Part model, mm, in its own coordinate system. Face numbers are marked on the shaded views. A direction names the side the tool comes from. Round coordinates to 2 decimals unless told otherwise and drop trailing zeros. Loops run counter-clockwise (first coordinate to the right, second up) from the corner with the lowest first, then second, coordinate; pieces in that order, holes last. Notation, with made-up numbers: (86, 89) -> (141, 89) arc R10 cw to (141, 98) -> close; hole circle Ø5 at (48, 74). An arc over 180 degrees is marked (long way). Answer as CSV lines item,"result".
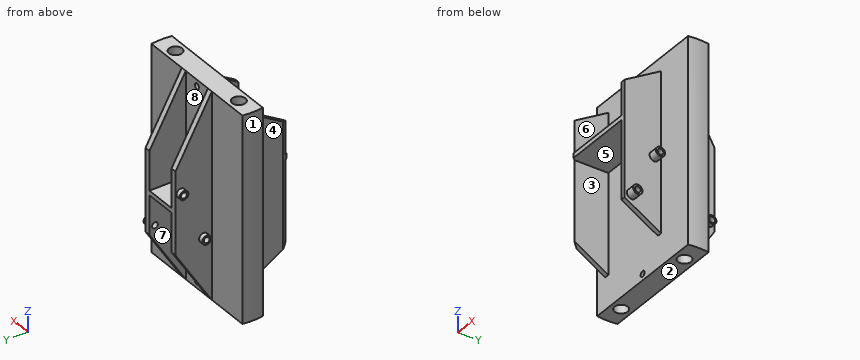
from build123d import *

# Parameters (mm, degrees)
SKETCH1_R            = 5.715
SKETCH1_R_2          = 3.683
BOSS_EXTRUDE2_DEPTH  = 114.3
SKETCH2_W            = 3.175
SKETCH2_H            = 45.974
BOSS_EXTRUDE3_DEPTH  = 20.32
SKETCH8_W            = 17.78
SKETCH8_H            = 2.54
BOSS_EXTRUDE6_DEPTH  = 20.32
BOSS_EXTRUDE9_DEPTH  = 20.32
CUT_EXTRUDE5_REACH   = 130.614
SKETCH10_R           = 1.5875
CUT_EXTRUDE6_REACH   = 126.596
SKETCH13_R           = 1.5875
BOSS_EXTRUDE14_DEPTH = 3.175
BOSS_EXTRUDE15_DEPTH = 3.175
BOSS_EXTRUDE16_START = 5.08
SKETCH12_R           = 2.590347575
SKETCH12_R_2         = 1.5875
SKETCH12_R_3         = 2.612210891
BOSS_EXTRUDE16_DEPTH = 5.08
CHAMFER1_SIZE        = 2.54
SKETCH21_R           = 1.6256
CUT_EXTRUDE7_DEPTH   = 5.08
SKETCH22_R           = 1.6256
CUT_EXTRUDE8_DEPTH   = 5.08
BOSS_EXTRUDE17_START = 2.54
SKETCH23_R           = 2.426614549
SKETCH23_R_2         = 1.6256
SKETCH23_R_3         = 2.598483989
BOSS_EXTRUDE17_DEPTH = 2.54
BOSS_EXTRUDE18_START = 2.54
SKETCH24_R           = 2.467964506
SKETCH24_R_2         = 1.6256
SKETCH24_R_3         = 2.533270714
BOSS_EXTRUDE18_DEPTH = 2.54
SKETCH25_R           = 48.771557558
SKETCH25_R_2         = 36.957
CUT_EXTRUDE9_DEPTH   = 124.263624906
CUT_EXTRUDE10_DEPTH  = 129.148442846


with BuildPart() as part:
    # Sketch1 → Boss-Extrude2 (new body)
    # profile 1 of 8: a face of its own
    with BuildSketch(Plane.XY):
        with BuildLine():
            Line((25.4, 5.715), (-25.4, 5.715))
            ThreePointArc((-25.4, 5.715), (-21.358884746, 4.041115254), (-19.685, 0))
            Line((-19.685, 0), (19.685, 0))
            ThreePointArc((19.685, 0), (21.358884746, 4.041115254), (25.4, 5.715))
        make_face()
    # profile 2 of 8: a face of its own
    with BuildSketch(Plane.XY):
        with Locations((-25.4, 0)):
            Circle(SKETCH1_R)
        with Locations((-25.4, 0)):
            Circle(SKETCH1_R_2, mode=Mode.SUBTRACT)
    # profile 3 of 8: a face of its own
    with BuildSketch(Plane.XY):
        with Locations((25.4, 0)):
            Circle(SKETCH1_R)
        with Locations((25.4, 0)):
            Circle(SKETCH1_R_2, mode=Mode.SUBTRACT)
    # profile 4 of 8: a face of its own
    with BuildSketch(Plane.XY):
        with BuildLine():
            ThreePointArc((-31.115, 0), (-29.441115254, 4.041115254), (-25.4, 5.715))
            Line((-25.4, 5.715), (-37.668936473, 5.715))
            ThreePointArc((-37.668936473, 5.715), (-37.992081278, 2.865616895), (-38.1, 0))
            Line((-38.1, 0), (-31.115, 0))
        make_face()
    # profile 5 of 8: a face of its own
    with BuildSketch(Plane.XY):
        with BuildLine():
            Line((37.668936473, 5.715), (25.4, 5.715))
            ThreePointArc((25.4, 5.715), (29.441115254, 4.041115254), (31.115, 0))
            Line((31.115, 0), (38.1, 0))
            ThreePointArc((38.1, 0), (37.992081278, 2.865616895), (37.668936473, 5.715))
        make_face()
    # profile 6 of 8: a face of its own
    with BuildSketch(Plane.XY):
        with BuildLine():
            Line((38.1, 0), (31.115, 0))
            ThreePointArc((31.115, 0), (29.441115254, -4.041115254), (25.4, -5.715))
            Line((25.4, -5.715), (37.668936473, -5.715))
            ThreePointArc((37.668936473, -5.715), (37.992081278, -2.865616895), (38.1, 0))
        make_face()
    # profile 7 of 8: a face of its own
    with BuildSketch(Plane.XY):
        with BuildLine():
            Line((19.685, 0), (-19.685, 0))
            ThreePointArc((-19.685, 0), (-21.358884746, -4.041115254), (-25.4, -5.715))
            Line((-25.4, -5.715), (25.4, -5.715))
            ThreePointArc((25.4, -5.715), (21.358884746, -4.041115254), (19.685, 0))
        make_face()
    # profile 8 of 8: a face of its own
    with BuildSketch(Plane.XY):
        with BuildLine():
            ThreePointArc((-25.4, -5.715), (-29.441115254, -4.041115254), (-31.115, 0))
            Line((-31.115, 0), (-38.1, 0))
            ThreePointArc((-38.1, 0), (-37.992081278, -2.865616895), (-37.668936473, -5.715))
            Line((-37.668936473, -5.715), (-25.4, -5.715))
        make_face()
    extrude(amount=BOSS_EXTRUDE2_DEPTH)

    # Sketch2 → Boss-Extrude3 (add)
    with BuildSketch(Plane(origin=(0, 5.715, 0), x_dir=(1, 0, 0), z_dir=(0, 1, 0))):
        with Locations((-10.427436473, -54.991)):
            Rectangle(SKETCH2_W, SKETCH2_H)
        with Locations((10.527563527, -54.991)):
            Rectangle(SKETCH2_W, SKETCH2_H)
    extrude(amount=BOSS_EXTRUDE3_DEPTH)

    # Sketch8 → Boss-Extrude6 (add)
    with BuildSketch(Plane(origin=(0, 5.715, 0), x_dir=(1, 0, 0), z_dir=(0, 1, 0))):
        with Locations((0.050063527, -54.991)):
            Rectangle(SKETCH8_W, SKETCH8_H)
    extrude(amount=BOSS_EXTRUDE6_DEPTH)

    # Sketch9 → Boss-Extrude9 (add)
    with BuildSketch(Plane.XZ.offset(5.715)):
        Polygon((12.268936473, 73.66), (12.268936473, 17.78), (14.808936473, 17.78), (14.808936473, 106.68), (12.268936473, 106.68), (12.268936473, 76.2), (-27.508936473, 76.2), (-27.508936473, 106.68), (-30.048936473, 106.68), (-30.048936473, 17.78), (-27.508936473, 17.78), (-27.508936473, 73.66), align=None)
    extrude(amount=BOSS_EXTRUDE9_DEPTH)

    # Sketch10 → Cut-Extrude5 (cut, up to next)
    with BuildSketch(Plane(origin=(14.808936473, 0, 0), x_dir=(0, 0, -1), z_dir=(1, 0, 0)), mode=Mode.PRIVATE) as cut_extrude5_sk1:
        with Locations((-58.42, -9.525)):
            Circle(SKETCH10_R)
    cut_extrude5_tool1 = extrude(cut_extrude5_sk1.sketch, amount=-CUT_EXTRUDE5_REACH, mode=Mode.PRIVATE) & part.part
    # Sketch10 → Cut-Extrude5 (cut, up to next)
    with BuildSketch(Plane(origin=(14.808936473, 0, 0), x_dir=(0, 0, -1), z_dir=(1, 0, 0)), mode=Mode.PRIVATE) as cut_extrude5_sk2:
        with Locations((-33.02, -22.225)):
            Circle(SKETCH10_R)
    cut_extrude5_tool2 = extrude(cut_extrude5_sk2.sketch, amount=-CUT_EXTRUDE5_REACH, mode=Mode.PRIVATE) & part.part
    add(cut_extrude5_tool1.solids().sort_by_distance((14.808936, -9.525, 58.42))[0], mode=Mode.SUBTRACT)
    add(cut_extrude5_tool2.solids().sort_by_distance((14.808936, -22.225, 33.02))[0], mode=Mode.SUBTRACT)

    # Sketch13 → Cut-Extrude6 (cut, up to next)
    with BuildSketch(Plane.XZ.offset(5.715), mode=Mode.PRIVATE) as cut_extrude6_sk1:
        with Locations(Location((0, 110.744, 0), (0, 0, 270))):
            Circle(SKETCH13_R)
    cut_extrude6_tool1 = extrude(cut_extrude6_sk1.sketch, amount=-CUT_EXTRUDE6_REACH, mode=Mode.PRIVATE) & part.part
    # Sketch13 → Cut-Extrude6 (cut, up to next)
    with BuildSketch(Plane.XZ.offset(5.715), mode=Mode.PRIVATE) as cut_extrude6_sk2:
        with Locations(Location((0, 3.556, 0), (0, 0, 270))):
            Circle(SKETCH13_R)
    cut_extrude6_tool2 = extrude(cut_extrude6_sk2.sketch, amount=-CUT_EXTRUDE6_REACH, mode=Mode.PRIVATE) & part.part
    add(cut_extrude6_tool1.solids().sort_by_distance((0, -5.715, 110.744))[0], mode=Mode.SUBTRACT)
    add(cut_extrude6_tool2.solids().sort_by_distance((0, -5.715, 3.556))[0], mode=Mode.SUBTRACT)

    # Sketch18 → Boss-Extrude14 (add)
    with BuildSketch(Plane.ZY.offset(12.014936473)):
        Polygon((77.978, 5.715), (77.978, 26.035), (114.3, 5.715), align=None)
        Polygon((32.004, 26.035), (32.004, 5.715), (0, 5.715), align=None)
    extrude(amount=-BOSS_EXTRUDE14_DEPTH)

    # Sketch19 → Boss-Extrude15 (add)
    with BuildSketch(Plane(origin=(12.115063527, 0, 0), x_dir=(0, 0, -1), z_dir=(1, 0, 0))):
        Polygon((-32.004, 26.035), (0, 5.715), (-32.004, 5.715), align=None)
        Polygon((-77.978, 5.715), (-114.3, 5.715), (-77.978, 26.035), align=None)
    extrude(amount=-BOSS_EXTRUDE15_DEPTH)

    # Sketch12 → Boss-Extrude16 (add)
    # profile 1 of 2: a face of its own
    with BuildSketch(Plane(origin=(14.808936473, 0, 0), x_dir=(0, 0, -1), z_dir=(1, 0, 0)).offset(BOSS_EXTRUDE16_START)):
        with Locations(Location((-58.42, -9.525, 0), (0, 0, 180))):
            Circle(SKETCH12_R)
        with Locations((-58.42, -9.525)):
            Circle(SKETCH12_R_2, mode=Mode.SUBTRACT)
    # profile 2 of 2: a face of its own
    with BuildSketch(Plane(origin=(14.808936473, 0, 0), x_dir=(0, 0, -1), z_dir=(1, 0, 0)).offset(BOSS_EXTRUDE16_START)):
        with Locations(Location((-33.02, -22.225, 0), (0, 0, 180))):
            Circle(SKETCH12_R_3)
        with Locations((-33.02, -22.225)):
            Circle(SKETCH12_R_2, mode=Mode.SUBTRACT)
    extrude(amount=-BOSS_EXTRUDE16_DEPTH)

    # Chamfer1
    chamfer1_edges = [part.edges().sort_by_distance(p)[0] for p in [
        (-30.048936473, -26.035, 62.23),
    ]]
    chamfer(chamfer1_edges, length=CHAMFER1_SIZE)

    # Sketch21 → Cut-Extrude7 (cut)
    with BuildSketch(Plane.ZY.offset(12.014936473)):
        with Locations((65.125187458, 23.037602192)):
            Circle(SKETCH21_R)
        with Locations((35.915187458, 10.337602192)):
            Circle(SKETCH21_R)
    extrude(amount=-CUT_EXTRUDE7_DEPTH, mode=Mode.SUBTRACT)

    # Sketch22 → Cut-Extrude8 (cut)
    with BuildSketch(Plane(origin=(12.115063527, 0, 0), x_dir=(0, 0, -1), z_dir=(1, 0, 0))):
        with Locations((-36.092684175, 22.91159358)):
            Circle(SKETCH22_R)
        with Locations((-65.302684175, 10.21159358)):
            Circle(SKETCH22_R)
    extrude(amount=-CUT_EXTRUDE8_DEPTH, mode=Mode.SUBTRACT)

    # Sketch23 → Boss-Extrude17 (add)
    # profile 1 of 2: a face of its own
    with BuildSketch(Plane(origin=(12.115063527, 0, 0), x_dir=(0, 0, -1), z_dir=(1, 0, 0)).offset(BOSS_EXTRUDE17_START)):
        with Locations(Location((-36.092684175, 22.91159358, 0), (0, 0, 180))):
            Circle(SKETCH23_R)
        with Locations((-36.092684175, 22.91159358)):
            Circle(SKETCH23_R_2, mode=Mode.SUBTRACT)
    # profile 2 of 2: a face of its own
    with BuildSketch(Plane(origin=(12.115063527, 0, 0), x_dir=(0, 0, -1), z_dir=(1, 0, 0)).offset(BOSS_EXTRUDE17_START)):
        with Locations(Location((-65.302684175, 10.21159358, 0), (0, 0, 180))):
            Circle(SKETCH23_R_3)
        with Locations((-65.302684175, 10.21159358)):
            Circle(SKETCH23_R_2, mode=Mode.SUBTRACT)
    extrude(amount=-BOSS_EXTRUDE17_DEPTH)

    # Sketch24 → Boss-Extrude18 (add)
    # profile 1 of 2: a face of its own
    with BuildSketch(Plane.ZY.offset(12.014936473).offset(BOSS_EXTRUDE18_START)):
        with Locations(Location((65.125187458, 23.037602192, 0), (0, 0, 180))):
            Circle(SKETCH24_R)
        with Locations((65.125187458, 23.037602192)):
            Circle(SKETCH24_R_2, mode=Mode.SUBTRACT)
    # profile 2 of 2: a face of its own
    with BuildSketch(Plane.ZY.offset(12.014936473).offset(BOSS_EXTRUDE18_START)):
        with Locations(Location((35.915187458, 10.337602192, 0), (0, 0, 180))):
            Circle(SKETCH24_R_3)
        with Locations((35.915187458, 10.337602192)):
            Circle(SKETCH24_R_2, mode=Mode.SUBTRACT)
    extrude(amount=-BOSS_EXTRUDE18_DEPTH)

    # Sketch25 → Cut-Extrude9 (cut, through all)
    with BuildSketch(Plane(origin=(0, 0, 0), x_dir=(-1, 0, 0), z_dir=(0, 0, -1))):
        Circle(SKETCH25_R)
        Circle(SKETCH25_R_2, mode=Mode.SUBTRACT)
    extrude(amount=-CUT_EXTRUDE9_DEPTH, mode=Mode.SUBTRACT)

    # Sketch26 → Cut-Extrude10 (cut, through all)
    with BuildSketch(Plane(origin=(14.808936473, 0, 0), x_dir=(0, 0, -1), z_dir=(1, 0, 0))):
        Polygon((-29.972, -26.035), (-17.78, -5.715), (-17.78, -26.035), align=None)
        Polygon((-106.68, -5.715), (-106.68, -26.035), (-94.488, -26.035), align=None)
    extrude(amount=-CUT_EXTRUDE10_DEPTH, mode=Mode.SUBTRACT)


solid = part.part
Q1. Saw through at A-A, the plane y = 0. Write the cut outline in (x, z) (1 decimal), then the cut area to 3 significant figures.
Geometry results:
outline,"(-37, 0) -> (-29.1, 0) -> (-29.1, 114.3) -> (-37, 114.3) -> close; (-21.7, 0) -> (21.7, 0) -> (21.7, 114.3) -> (-21.7, 114.3) -> close; (29.1, 0) -> (37, 0) -> (37, 114.3) -> (29.1, 114.3) -> close; hole circle Ø3.2 at (0, 3.6); hole circle Ø3.2 at (0, 110.7)"
area,"6,750 mm2"
Q2. Saw through at B-B, the plane z = 58.42. Give the number of separate pieces and of enclosed holes in the cut face, then the cut area to 3 significant figures.
Geometry results:
separate pieces,"2"
enclosed holes,"2"
area,"983 mm2"
Q3. Two-plate mould, pull along X, no slides. Class the marked faces 1, 2 and 3: pulls with the +X half, pulls with the -X half, needs draft (parallel to the pull), parting line crosses it, or undercut.
Geometry results:
face 1,"pulls with the -X half"
face 2,"needs draft"
face 3,"undercut"
Q4. Saw through at D-D, the plane x = 0. Write the cut outline in (y, z) (1 decimal), then the cut area to 3 significant figures.
Geometry results:
outline,"(-26, 73.7) -> (-5.7, 73.7) -> (-5.7, 5.1) -> (5.7, 5.1) -> (5.7, 53.7) -> (26, 53.7) -> (26, 56.3) -> (5.7, 56.3) -> (5.7, 109.2) -> (-5.7, 109.2) -> (-5.7, 76.2) -> (-26, 76.2) -> close; (-5.7, 0) -> (5.7, 0) -> (5.7, 2) -> (-5.7, 2) -> close; (-5.7, 112.3) -> (5.7, 112.3) -> (5.7, 114.3) -> (-5.7, 114.3) -> close"
area,"1,340 mm2"
Q5. Saw through at C-C, the plane x = 25.4. Write the cut outline in (y, z) (3 decimals).
Geometry results:
outline,"(-5.715, 0) -> (-3.683, 0) -> (-3.683, 114.3) -> (-5.715, 114.3) -> close; (3.683, 0) -> (5.715, 0) -> (5.715, 114.3) -> (3.683, 114.3) -> close"
Q6. Drop flat-ended pins along their axis: P1, Ø2.5, axis at y = -21.5, z = 33, coming from the +X side; P2, Ø5, axis at y = 10.34, z = 35.92, coming from the +X side; P3, Ø6, axis at x = -4.5, z = 35.5, coming from the +Y side (3 decimals). Give the stop position or say it passes through.
Geometry results:
P1,"x = 19.89"
P2,"x = 12.12"
P3,"y = 5.715"
Q7. Drill centre lines: line 1 along Y through (x, z) = (17, 33.02) (1 decimal); line 2 along X through (y, z) = (-9, 73.5); line 3 along X through (y, z) = (21, 73.5). Where is each one in solid material? Low to high.
Geometry results:
line 1,"-24.8 to -23.8, -20.6 to -19.6, -5.7 to 5.7"
line 2,"-30.05 to -27.51, 12.27 to 14.81"
line 3,"-12.01 to -8.84, 8.94 to 12.12"
Q8. Which spindle directions (+Z, -Z, +X, -X, +Y, -Y) get a long thin tool onto all of the face, cutting with end or side? Do the marked faces 4, 5, 6, 7 and 8. Say none if no direction does.
Geometry results:
face 4,"+Z, -Z, -X, -Y"
face 5,"-Z, -Y"
face 6,"+Z, -Y"
face 7,"-Z, +Y"
face 8,"+Z, +Y"
